Autodesk Inventor part; units mm, degrees
ref_plane "YZ Plane" through (0, 0, 0) normal (1, 0, 0) x (0, 1, 0)
ref_plane "XZ Plane" through (0, 0, 0) normal (0, 1, 0) x (-1, 0, 0)
ref_plane "XY Plane" through (0, 0, 0) normal (0, 0, 1) x (1, 0, 0)
sketch "Sketch1" plane through (0, 0, 0) normal (0, 1, 0) x (-1, 0, 0)
  circle A0 centre (0, 0) radius 85
  dimension "d0" = 170
extrude "Extrusion1" add sketch "Sketch1" along normal blind 180
shell "Shell1" thickness 2 removed faces 1 at (4.1372, 180, 51.3099)
sketch "Sketch2" plane through (0, 0, 0) normal (1, 0, 0) x (0, 1, 0)
  line L0 (180, -85) -> (180, 85)
  line L1 (0, 85) -> (0, -85)
  arc A0 (180, -85) -> (180, 85) centre (180, 0) ccw
  line L2 (0, 85) -> (180, 85)
  line L3 (0, -85) -> (180, -85)
  arc A1 (180, -81) -> (180, 81) centre (180, 0) ccw
  point P0 (0, 0)
  dimension "d4" = 4
extrude "Extrusion2" add sketch "Sketch2" along normal mid plane 4 contours L0 A1 A0
properties part number "emmer"
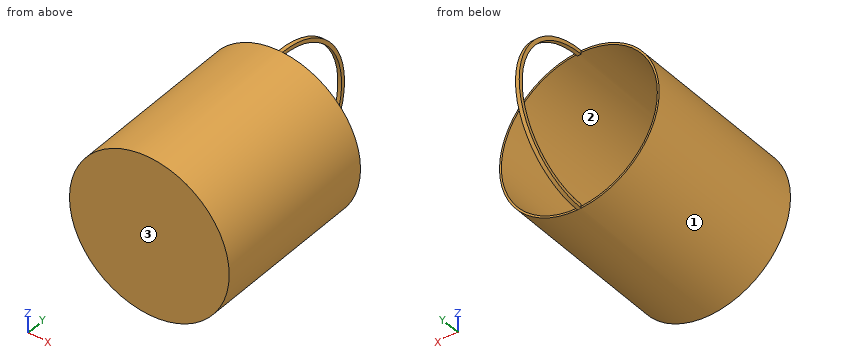
Check sheet for the modelled part. Datum: model origin and axes. Units: mm. Face numbers are marked on the shaded views. Round coordinates to 2 decimals unless told otherwise and drop trailing zeros. Order: outer loops, then holes, each group sorted by start corner. A loop starts at its lowest first (then second) coordinate and runs counter-clockwise, first axis right, second up. Notation, with made-up numbers: M -19.75,29 L 20.25,29 A22 cw 20.25,44 Z; hole C -27.75,42 d6. An arc over 180 degrees is marked long. One line per item, written item: value. Start each with the question number.
1. Section check B-B on y = 234.5. Enter the section's corners in (x, z).
2. Gauge pin test, flat ends, axial feed: P1, Ø10, axis at x = -39, z = 43, coming from the +Y side; P2, Ø2, axis at y = 162.5, z = 59.5, coming from the -X side; P3, Ø5, axis at x = 22, y = 78.5, coming from the -Z side. Record the tip position at first contact, or that the pin passes through.
3. Release check for a two-part mould opening along Z. For the marked faces 1, 2 and 3 record: released by +Z, released by -Z, zero draft, split by the parting line, or undercut.
4. Section check A-A on z = 0. Enter the section's corners in (x, y).
5. Section check C-C on y = 93. Enter the section's corners in (x, z), and give its area (3 significant figures).
6. Section check D-D on z = -18. Enter the section's corners in (x, y), and give its area (3 significant figures).
7. Scan lines: line 1 along Z through (x, y) = (0, 52); line 2 along Y through (x, z) = (31, -17.5). Record each from-to range of solid material in increasing order.
Results found:
1. outline: M -2,-65.23 L 2,-65.23 L 2,-59.92 L -2,-59.92 Z; M -2,59.92 L 2,59.92 L 2,65.23 L -2,65.23 Z
2. P1: y = 2
2. P2: x = -61.67
2. P3: z = -82.73
3. face 1: split by the parting line
3. face 2: undercut
3. face 3: zero draft
4. outline: M -85,0 L 85,0 L 85,180 L 83,180 L 83,2 L -83,2 L -83,180 L -85,180 Z; M -2,261 L 2,261 L 2,265 L -2,265 Z
5. outline: C 0,0 d170; hole C 0,0 d166
5. area: 1,060 mm^2
6. outline: M -83.07,0 L 83.07,0 L 83.07,180 L 81.02,180 L 81.02,2 L -81.02,2 L -81.02,180 L -83.07,180 Z; M -2,258.97 L 2,258.97 L 2,263.07 L -2,263.07 Z
6. area: 1,080 mm^2
7. line 1: -85 to -83, 83 to 85
7. line 2: 0 to 2
